Check sheet for the modelled part. Datum: model origin and axes. Units: mm. Face numbers are marked on the shaded views. A direction names the side the tool comes from. Round coordinates to 2 decimals unless told otherwise and drop trailing zeros. Write each loop counter-clockwise with the first axis right and the second up, starting at its lowest first coordinate (ties: lowest second). Pieces come first, ordered by that corner, then holes. Notation, with made-up numbers: (-4, 10.5) -> (22, 10.5) arc R17 cw to (22, 34.5) -> close; hole circle Ø9 at (41.5, 62.25). An arc over 180 degrees is marked (long way). One line per item, written item: value.
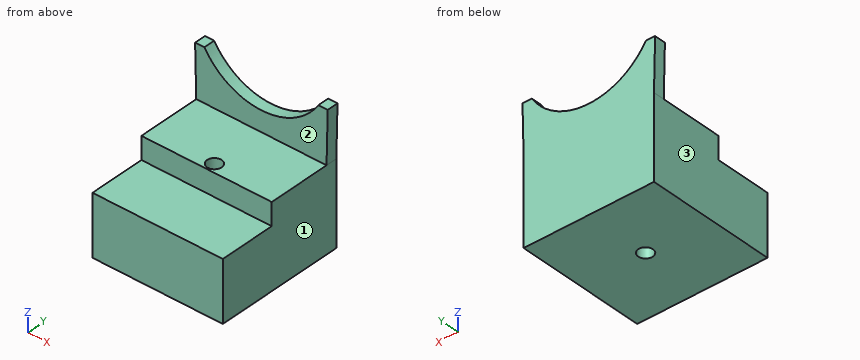
Autodesk Inventor part; units mm, degrees
ref_plane "YZ Plane" through (0, 0, 0) normal (1, 0, 0) x (0, 1, 0)
ref_plane "XZ Plane" through (0, 0, 0) normal (0, 1, 0) x (-1, 0, 0)
ref_plane "XY Plane" through (0, 0, 0) normal (0, 0, 1) x (1, 0, 0)
sketch "Sketch1" plane through (0, 0, 0) normal (0, 0, 1) x (1, 0, 0)
  line L0 (29, -29) -> (-29, -29)
  line L1 (-29, -29) -> (-29, 29)
  line L2 (-29, 29) -> (29, 29)
  line L3 (29, 29) -> (29, -29)
  line L4 (29, -29) -> (-29, 29) construction
  line L5 (-29, -29) -> (29, 29) construction
  point P0 (0, 0)
  point P1 (0, 0)
  dimension "d0" = 58
  dimension "d1" = 58
extrude "Extrusion1" add sketch "Sketch1" along normal blind 36.866
sketch "Sketch2" plane through (0, 0, 36.866) normal (0, 0, 1) x (1, 0, 0)
  line L0 (-29, 29) -> (-29, -29)
  line L1 (29, -29) -> (29, 29)
  line L2 (-29, -4) -> (29, -4)
  line L3 (29, -4) -> (29, -29)
  line L4 (29, -29) -> (-29, -29)
  line L5 (-29, -29) -> (-29, -4)
  point P0 (0, 0)
extrude "Extrusion2" cut sketch "Sketch2" against normal blind 10
hole "Hole1" at (0, 0, 0) direction (0, 0, 1) diameter 6.5 end through all
sketch "Sketch3" plane through (-29, 29, 0) normal (0, 1, 0) x (1, 0, 0)
  line L0 (0, 0) -> (58, 0)
  line L1 (0, 0) -> (0, -36.866)
  line L2 (58, -36.866) -> (0, -36.866)
  line L3 (58, 0) -> (58, -36.866)
  arc A0 (3.645, -60) -> (54.355, -60) centre (29, -75.8) ccw
  line L4 (58, -36.866) -> (58, -26.866)
  line L5 (58, -36.866) -> (58.8673, -75.1229)
  line L6 (0, -26.866) -> (0, -36.866)
  line L7 (0, -36.866) -> (-0.8673, -76.4771)
  line L8 (58.5245, -60) -> (-0.5065, -60)
  arc A1 (54.355, -60) -> (3.645, -60) centre (29, -75.8) ccw
  point P0 (29, 0)
  dimension "d13" = 59.75
extrude "Extrusion3" add sketch "Sketch3" against normal blind 5 contours L2 L5 L8 A1 L7
properties part number "Iris15-mount"
Item 1: Sectioned sample at B-B (y = 0). Enter the section's corners in (x, z), then the cut area to 3 significant figures.
Result set:
outline: (-29, 0) -> (-3.25, 0) -> (-3.25, 36.87) -> (-29, 36.87) -> close; (3.25, 0) -> (29, 0) -> (29, 36.87) -> (3.25, 36.87) -> close
area: 1,900 mm^2
Item 2: Sectioned sample at C-C (z = 31). Enter the section's corners in (x, y), then the cut area to 3 significant figures.
Result set:
outline: (-29, -4) -> (29, -4) -> (29, 29) -> (-29, 29) -> close; hole circle Ø6.5 at (0, 0)
area: 1,880 mm^2
Item 3: Material ranges on line 1 along Y through (x, z) = (0, 29); line 2 along X through (y, z) = (0, 28.5), recorded low to high.
Result set:
line 1: -4 to -3.25, 3.25 to 29
line 2: -29 to -3.25, 3.25 to 29
Item 4: Tool access check on the marked faces 1, 2 and 3. Record the directions out of +Z, -Z, +X, -X, +Y, -Y that give a thin tool (end or side, any length) a straight path to the whole face; none if there is none.
Result set:
face 1: -Z, +X, +Y, -Y
face 2: +Z, +X, -X, -Y
face 3: -Z, -X, +Y, -Y
Item 5: Depth check by flat-ended pin: pin 1 (11 mm diameter, centred on y = -13.5, z = 26.5, fed in from +X); pin 2 (10.5 mm diameter, centred on x = 0, y = 0, fed in from +Z); pin 3 (8 mm diameter, centred on x = -10.5, y = -2, fed in from -Z); pin 4 (18.5 mm diameter, centred on x = 7.5, z = 45, fed in from -Y). Enter the tip coordinate at first touch or a pass-through.
Result set:
pin 1: x = 29
pin 2: z = 36.87
pin 3: z = 0
pin 4: y = -4
Item 6: Sectioned sample at A-A (x = 0). Enter the section's corners in (y, z) (3 decimals), then the cut area to 3 significant figures.
Result set:
outline: (-29, 0) -> (-3.25, 0) -> (-3.25, 36.866) -> (-4, 36.866) -> (-4, 26.866) -> (-29, 26.866) -> close; (3.25, 0) -> (29, 0) -> (29, 45.925) -> (24, 45.925) -> (24, 36.866) -> (3.25, 36.866) -> close
area: 1,690 mm^2
Item 7: Sectioned sample at D-D (x = 14.5). Enter the section's corners in (y, z).
Result set:
outline: (-29, 0) -> (29, 0) -> (29, 49.68) -> (24, 49.68) -> (24, 36.87) -> (-4, 36.87) -> (-4, 26.87) -> (-29, 26.87) -> close
